Input: part model. Units: mm. Frame: model coordinates. A direction names the side the tool comes from. Give positions to 0.01 mm unless a question says otherwise; leave off trailing zeros. Loops run counter-clockwise (first coordinate to the right, second up) from the corner with the lowest first, then second, coordinate; pieces in that order, holes last. Notation, with made-up numbers: (-15, 48.25) -> (36, 48.25) arc R29 ccw to (36, 84.25) -> close; hole circle Ø5 at (-6.5, -0.75). An arc over 180 degrees is marked (long way). Answer as a JSON object with one key per item and string values. Group by question number.
Autodesk Fusion 360 part; units mm, degrees
sketch "Sketch1" plane through (0, 0, 0) normal (0, 0, 1) x (1, 0, 0)
  line L0 (0, 0) -> (26, 0)
  line L1 (26, 0) -> (26, 26)
  line L2 (26, 26) -> (0, 26)
  line L3 (0, 26) -> (0, 0)
  dimension "d1" = 26
  dimension "d2" = 26
extrude "Extrude1" add sketch "Sketch1" along normal blind 2
sketch "Sketch2" plane through (0, 0, 2) normal (0, 0, 1) x (-1, 0, 0)
  line L0 (0, -26) -> (0, 0)
  line L1 (0, 0) -> (-26, 0)
  line L2 (-26, 0) -> (-26, -26)
  line L3 (-26, -26) -> (0, -26)
  line L4 (-2, -24) -> (-24, -24)
  line L5 (-24, -24) -> (-24, -2)
  line L6 (-24, -2) -> (-2, -2)
  line L7 (-2, -2) -> (-2, -24)
extrude "Extrude2" add sketch "Sketch2" along normal blind 1.5
extrude "Extrude3" add 1 faces at (0.6667, 9.3333, 3.5) along direction (0, 0, 1) blind 2
extrude "Extrude4" add 1 faces at (9.3333, 16.6667, 2) along direction (0, 0, 1) blind 2
extrude "Extrude5" cut 1 faces at (0.6667, 9.3333, 5.5) along direction (0, 0, -1) blind 0.5
fillet "Fillet1" radius 3 4 edges at (0, 26, 2.5) (26, 26, 2.5) (0, 0, 2.5) (26, 0, 2.5)
fillet "Fillet2" radius 1 16 edges at (0, 13, 5) (0.8787, 25.1213, 5) (13, 26, 5) (25.1213, 25.1213, 5) (26, 13, 5) (25.1213, 0.8787, 5) (13, 0, 5) (0.8787, 0.8787, 5) (26, 13, 0) (25.1213, 25.1213, 0) (13, 26, 0) (0.8787, 25.1213, 0) (0, 13, 0) (0.8787, 0.8787, 0) (13, 0, 0) (25.1213, 0.8787, 0)
sketch "Sketch3" plane through (0, 0, 4) normal (0, 0, 1) x (-1, 0, 0)
  line L0 (-24, -2) -> (-24, -24)
  line L1 (-24, -24) -> (-2, -24)
  line L2 (-2, -24) -> (-2, -2)
  line L3 (-2, -2) -> (-24, -2)
  circle A0 centre (-7, -19) radius 1.5
  circle A1 centre (-19, -19) radius 1.5
  circle A2 centre (-19, -7) radius 1.5
  circle A3 centre (-7, -7) radius 1.5
  dimension "d16" = 3
  dimension "d17" = 3
  dimension "d18" = 3
  dimension "d19" = 3
extrude "Extrude6" cut sketch "Sketch3" against normal blind 4 contours A0 | A1 | A2 | A3
sketch "Sketch4" plane through (0, 0, 4) normal (0, 0, 1) x (-1, 0, 0)
  circle A0 centre (-7, -19) radius 1.5
  circle A1 centre (-7, -7) radius 1.5
  circle A2 centre (-19, -19) radius 1.5
  circle A3 centre (-19, -7) radius 1.5
  line L0 (-24, -2) -> (-24, -24)
  line L1 (-24, -24) -> (-2, -24)
  line L2 (-2, -24) -> (-2, -2)
  line L3 (-2, -2) -> (-24, -2)
  line L4 (-10.25, -20.8764) -> (-7, -22.7528)
  line L5 (-7, -22.7528) -> (-3.75, -20.8764)
  line L6 (-3.75, -20.8764) -> (-3.75, -17.1236)
  line L7 (-3.75, -17.1236) -> (-7, -15.2472)
  line L8 (-7, -15.2472) -> (-10.25, -17.1236)
  line L9 (-10.25, -17.1236) -> (-10.25, -20.8764)
  line L10 (-22.25, -20.8764) -> (-19, -22.7528)
  line L11 (-19, -22.7528) -> (-15.75, -20.8764)
  line L12 (-15.75, -20.8764) -> (-15.75, -17.1236)
  line L13 (-15.75, -17.1236) -> (-19, -15.2472)
  line L14 (-19, -15.2472) -> (-22.25, -17.1236)
  line L15 (-22.25, -17.1236) -> (-22.25, -20.8764)
  line L16 (-10.25, -8.8764) -> (-7, -10.7528)
  line L17 (-7, -10.7528) -> (-3.75, -8.8764)
  line L18 (-3.75, -8.8764) -> (-3.75, -5.1236)
  line L19 (-3.75, -5.1236) -> (-7, -3.2472)
  line L20 (-7, -3.2472) -> (-10.25, -5.1236)
  line L21 (-10.25, -5.1236) -> (-10.25, -8.8764)
  line L22 (-22.25, -8.8764) -> (-19, -10.7528)
  line L23 (-19, -10.7528) -> (-15.75, -8.8764)
  line L24 (-15.75, -8.8764) -> (-15.75, -5.1236)
  line L25 (-15.75, -5.1236) -> (-19, -3.2472)
  line L26 (-19, -3.2472) -> (-22.25, -5.1236)
  line L27 (-22.25, -5.1236) -> (-22.25, -8.8764)
  point P0 (-7, -19)
  point P1 (-19, -19)
  point P2 (-7, -7)
  point P3 (-19, -7)
  dimension "d22" = 3.25
  dimension "d23" = 3.25
  dimension "d24" = 3.25
  dimension "d25" = 3.25
extrude "Extrude7" cut sketch "Sketch4" against normal blind 2 contours L4 L5 L6 L7 L8 L9 | L10 L11 L12 L13 L14 L15 | L16 L17 L18 L19 L20 L21 | L22 L23 L24 L25 L26 L27
chamfer "Chamfer1" distance 0.5 angle 45 24 edges at (8.625, 4.1854, 4) (5.375, 4.1854, 4) (3.75, 7, 4) (5.375, 9.8146, 4) (8.625, 9.8146, 4) (10.25, 7, 4) (8.625, 16.1854, 4) (5.375, 16.1854, 4) (3.75, 19, 4) (5.375, 21.8146, 4) (8.625, 21.8146, 4) (10.25, 19, 4) (17.375, 21.8146, 4) (15.75, 19, 4) (17.375, 16.1854, 4) (20.625, 16.1854, 4) (22.25, 19, 4) (20.625, 21.8146, 4) (17.375, 9.8146, 4) (15.75, 7, 4) (17.375, 4.1854, 4) (20.625, 4.1854, 4) (22.25, 7, 4) (20.625, 9.8146, 4)
Q1. Section D-D on z = 0.4. Return the cut outline in (x, y).
Q2. Pull-direction query (X, two-part tool) for faces 3 (the face through (10.25, 19, 3)), 4 (the face through (12.86, 25.699, 4.715)), 5 (the face through (0.86, 0.9, 2.52)); classes: +X half, -X half, draft (parallel to the pull), parting line (faces both ways), or undercut.
Q3. Section A-A on y = 19. State how many separate pieces and enclosed holes the cut face has, then the cut area to 3 significant figures.
Q4. Pin query (flat end, axial travel): pin 1 Ø2 at (x, y) = (7.5, 8) entering from +Z; pin 2 Ø6 at (x, y) = (10, 14) entering from +Z; pin 3 Ø1.1 at (x, z) = (10, 4.5) entering from +Y; pin 4 Ø0.5 at (x, z) = (13, 4.5) entering from -Y. Return the tip coordinate at first contact, or that it passes through.
Q5. Ray query, probe 1 along Y at (x, z) = (19, 1.4); probe 2 along X at (y, z) = (6.75, 2.8). Return the intervals inside material, ascending.
Q6. Set-up query: faces 1 (the face through (12.8, 24, 4.5)), 2 (the face through (12.86, 25.715, 0.301)). Return all of +Z, -Z, +X, -X, +Y, -Y with unobstructed straight access to the full face (end or side cutting, diameter ignored); none if empty.
Numbers:
{
 "1": {"outline": "(0.2, 3) arc R2.8 ccw to (3, 0.2) -> (23, 0.2) arc R2.8 ccw to (25.8, 3) -> (25.8, 23) arc R2.8 ccw to (23, 25.8) -> (3, 25.8) arc R2.8 ccw to (0.2, 23) -> close; hole circle Ø3 at (7, 7); hole circle Ø3 at (7, 19); hole circle Ø3 at (19, 7); hole circle Ø3 at (19, 19)"},
 "2": {"face 3": "undercut", "face 4": "draft", "face 5": "-X half"},
 "3": {"separate pieces": "3", "enclosed holes": "0", "area": "68.6 mm²"},
 "4": {"pin 1": "stops at z = 2", "pin 2": "stops at z = 4", "pin 3": "stops at y = 26", "pin 4": "stops at y = 0.03"},
 "5": {"probe 1": "y = 0 to 5.5, 8.5 to 17.5, 20.5 to 26", "probe 2": "x = 0 to 3.75, 10.25 to 15.75, 22.25 to 26"},
 "6": {"face 1": "+Z", "face 2": "-Z, +X, -X, +Y"}
}
